Build history of the part. All positions in model axes, mm. Coordinates: 2 decimals unless noted, no trailing zeros. Loops run counter-clockwise (first coordinate to the right, second up) from the corner with the lowest first, then second, coordinate; pieces in that order, holes last.
(1) Slice it at A-A (y = -3). Give the cut face in (x, z).
(2) Two-plate mould, pull along Z, no slides. Class faces 1 (the face through (73.95, 31.892, -3.423)), 2 (the face through (150, -12, -1)), 3 (the face through (73.95, 39.325, -0.408)): pulls with the +Z half, pulls with the -Z half, needs draft (parallel to the pull), parting line crosses it, or undercut.
(3) Flat gauge pins, fed straight in: P1, Ø1.5, axis at x = 70, y = 14.5, coming from the -Z side; P2, Ø4, axis at x = 128, y = -33, coming from the -Z side; P3, Ø4, axis at x = 62.5, y = 37.5, coming from the -Z side. Where does each tip first touch, or does it go through?
(4) Wall check: L1, parallel to Z at x = 100, y = -24.5; L2, parallel to Z at x = 130, y = -14.5. Give the ranges that are in metal, low to high.
from build123d import *

# Parameters (mm, degrees)
F1_DEPTH = 150


with BuildPart() as f1:
    # F0 (on Right) → F1 (new body)
    with BuildSketch(Plane.YZ):
        Polygon((49.401502, -1.812943), (49.401429, -1.587792), (48.049564, -1.438415), (43.798746, -0.95), (40.948746, -0.609), (37.654746, -0.202), (33.954746, 0.266), (29.886746, 0.788), (25.497746, 1.356), (20.834746, 1.955), (15.948746, 2.564), (10.893746, 3.154), (5.723746, 3.699), (0.497746, 4.175), (-4.728254, 4.551), (-9.898254, 4.816), (-14.953254, 4.96), (-19.839254, 4.96), (-24.502254, 4.848), (-28.891254, 4.601), (-32.959254, 4.218), (-36.659254, 3.721), (-39.953254, 3.12), (-42.803254, 2.414), (-45.179254, 1.637), (-47.055254, 0.814), (-48.409254, -0.053), (-49.228254, -0.919), (-49.502254, -1.683), (-49.228254, -2.168), (-48.409254, -2.696), (-47.055254, -3.173), (-45.179254, -3.568), (-42.803254, -3.908), (-39.953254, -4.2), (-36.659254, -4.439), (-32.959254, -4.63), (-28.891254, -4.773), (-24.502254, -4.871), (-19.839254, -4.932), (-14.953254, -4.96), (-9.898254, -4.953), (-4.728254, -4.913), (0.497746, -4.84), (5.723746, -4.725), (10.893746, -4.568), (15.948746, -4.372), (20.834746, -4.137), (25.497746, -3.869), (29.886746, -3.576), (33.954746, -3.265), (37.654746, -2.951), (40.948746, -2.647), (43.798746, -2.366), (46.174746, -2.125), (48.046751, -1.944415), align=None)
    extrude(amount=F1_DEPTH)


solid = f1.part
Response values:
1. outline: (0, -4.89) - (150, -4.89) - (150, 4.43) - (0, 4.43) - close
2. face 1: pulls with the -Z half
2. face 2: needs draft
2. face 3: pulls with the +Z half
3. P1: stops at z = -4.46
3. P2: stops at z = -4.7
3. P3: stops at z = -3.13
4. L1: z = -4.87 to 4.85
4. L2: z = -4.96 to 4.95
